Geometry: see drawing. Coordinates: mm, zero at the bounding-box minimum. Round coordinates to 2 decimals unless told otherwise and drop trailing zeros. Write each loop counter-clockwise with the first axis right and the second up, starting at its lowest first coordinate (ties: lowest second). Pieces come first, ordered by that corner, then holes. Notation, with made-up numbers: M 49.25,-14 L 61.25,-14 A28 cw 61.25,21 Z; hole C -26,61.5 d4. An arc over 180 degrees is marked long. Use one line per item in the form item = value. Start each with the question number.
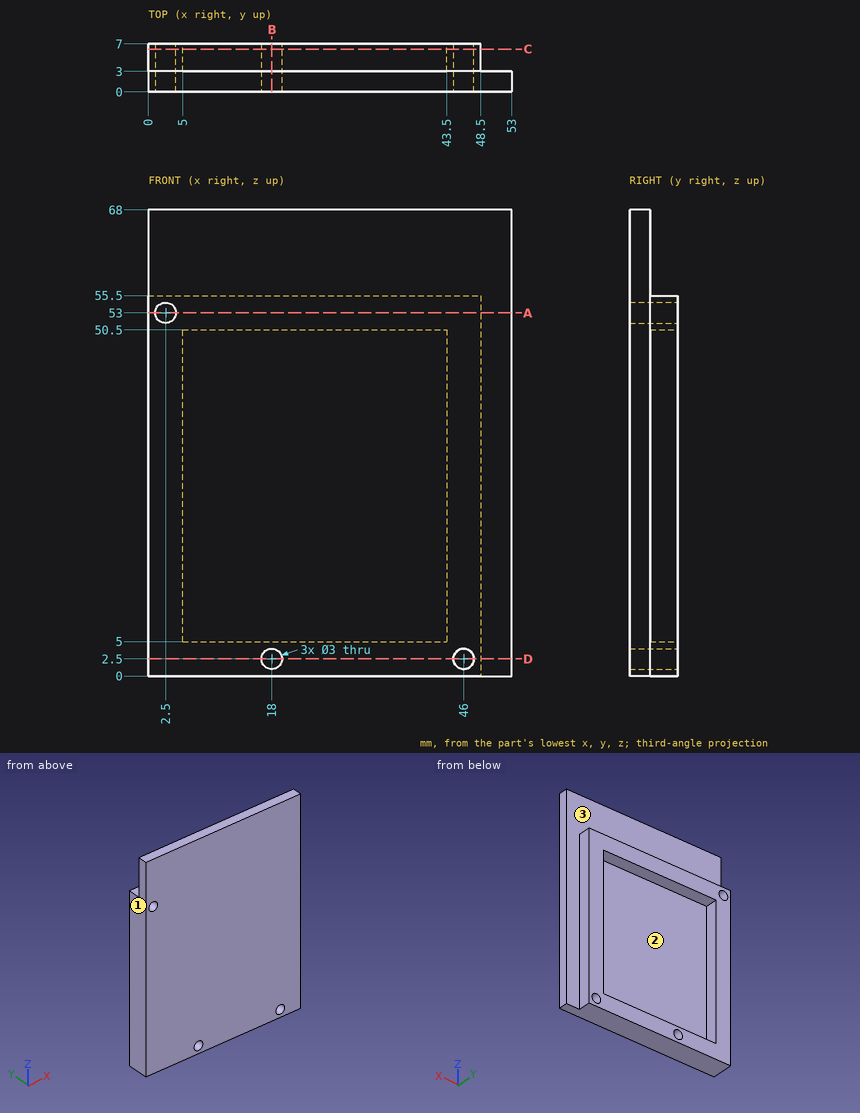
Item 1: Draft query along X for the marked faces 1, 2 and 3. Return one class per face: +X half, -X half, draft (parallel to the pull), parting line (faces both ways), or undercut.
Item 2: Cut plane D-D (z = 2.5). Output: boundary loops of the cut face in (x, y), plus the area to 3 significant figures.
Item 3: First-contact query: pin 1 (2 mm diameter, centred on x = 23, z = 9, fed in from +Y); pin 2 (1.2 mm diameter, centred on y = 6, z = 28.5, fed in from +X). Flat tips, straight axial feed; report the tip coordinate or a pass-through.
Item 4: Cut plane C-C (y = 6.25). Output: boundary loops of the cut face in (x, z), plus the area to 3 significant figures.
Item 5: Cut plane B-B (x = 18). Output: boundary loops of the cut face in (y, z), plus the area to 3 significant figures.
Item 6: Cut plane A-A (z = 53). Output: boundary loops of the cut face in (x, y).
Item 7: Ray query, line 1 (Z direction, x = 36, y = 3.75); line 2 (Z direction, x = 46, y = 2); line 3 (X direction, y = 5.25, z = 19.5). Return the intervals inside material, ascending. Write a range as from..to.
Final values:
q1.face_1 = -X half
q1.face_2 = undercut
q1.face_3 = draft
q2.outline = M 0,0 L 16.5,0 L 16.5,7 L 0,7 Z; M 19.5,0 L 44.5,0 L 44.5,7 L 19.5,7 Z; M 47.5,0 L 53,0 L 53,3 L 48.5,3 L 48.5,7 L 47.5,7 Z
q2.area = 311 mm^2
q3.pin_1 = 3
q3.pin_2 = 48.5
q4.outline = M 0,0 L 48.5,0 L 48.5,55.5 L 0,55.5 Z; hole C 2.5,53 d3; hole M 5,5 L 43.5,5 L 43.5,50.5 L 5,50.5 Z; hole C 18,2.5 d3; hole C 46,2.5 d3
q4.area = 919 mm^2
q5.outline = M 0,0 L 7,0 L 7,1 L 0,1 Z; M 0,4 L 7,4 L 7,5 L 3,5 L 3,50.5 L 7,50.5 L 7,55.5 L 3,55.5 L 3,68 L 0,68 Z
q5.area = 223 mm^2
q6.outline = M 0,0 L 1,0 L 1,7 L 0,7 Z; M 4,0 L 53,0 L 53,3 L 48.5,3 L 48.5,7 L 4,7 Z
q7.line_1 = 0..5, 50.5..55.5
q7.line_2 = 0..1, 4..68
q7.line_3 = 0..5, 43.5..48.5
